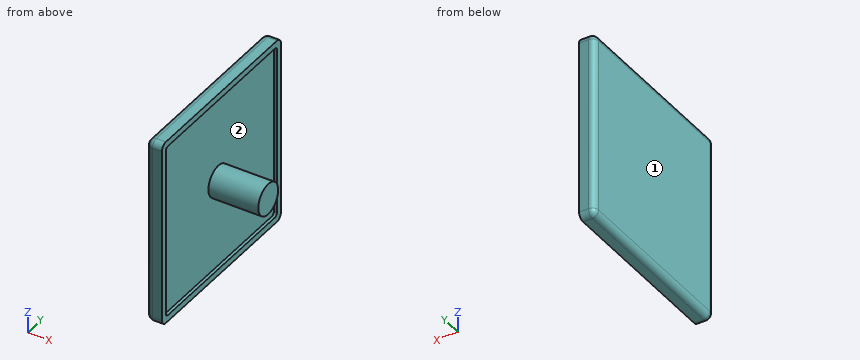
from build123d import *

# Parameters (mm, degrees)
SKETCH2_W           = 30
SKETCH2_H           = 30
BOSS_EXTRUDE1_DEPTH = 2.5
SKETCH3_W           = 28
SKETCH3_H           = 28
CUT_EXTRUDE1_DEPTH  = 0.5
FILLET1_R           = 1
FILLET2_R           = 1
FILLET3_R           = 0.5
SKETCH5_R           = 2.5
BOSS_EXTRUDE2_DEPTH = 8


with BuildPart() as part:
    # Sketch2 → Boss-Extrude1 (new body)
    with BuildSketch(Plane(origin=(0, 0, 0), x_dir=(0, 0, -1), z_dir=(1, 0, 0))):
        with Locations((15, 15)):
            Rectangle(SKETCH2_W, SKETCH2_H)
    extrude(amount=BOSS_EXTRUDE1_DEPTH)

    # Sketch3 → Cut-Extrude1 (cut)
    with BuildSketch(Plane(origin=(2.5, 0, 0), x_dir=(0, 0, -1), z_dir=(1, 0, 0))):
        with Locations((15, 15)):
            Rectangle(SKETCH3_W, SKETCH3_H)
    extrude(amount=-CUT_EXTRUDE1_DEPTH, mode=Mode.SUBTRACT)

    # Fillet1
    fillet1_edges = [part.edges().sort_by_distance(p)[0] for p in [
        (0, 30, -15),
        (0, 15, -30),
        (0, 0, -15),
        (0, 15, 0),
    ]]
    fillet(fillet1_edges, radius=FILLET1_R)

    # Fillet2
    # the kernel refuses this fillet: 1 mm, written as the material it takes off along each edge
    with BuildSketch(Plane(origin=(1, 29, -1), x_dir=(0, 1, 0), z_dir=(0, 0, 1))) as fillet2_piece_1_section:
        Polygon((0, 0), (FILLET2_R, 0), (FILLET2_R, FILLET2_R), (0, FILLET2_R), align=None)
    fillet2_piece_1 = extrude(amount=FILLET2_R, mode=Mode.PRIVATE)
    fillet2_piece_1 = fillet2_piece_1 - Plane(origin=(1, 29, -1), x_dir=(0.7071067811865475, -0.7071067811865475, 0), z_dir=(0, 0, 1)) * Sphere(FILLET2_R, mode=Mode.PRIVATE)
    add(fillet2_piece_1, mode=Mode.SUBTRACT)
    with BuildSketch(Plane(origin=(1, 29, -29), x_dir=(0, 1, 0), z_dir=(0, 0, -1))) as fillet2_piece_2_section:
        Polygon((0, 0), (FILLET2_R, 0), (FILLET2_R, -FILLET2_R), (0, -FILLET2_R), align=None)
    fillet2_piece_2 = extrude(amount=FILLET2_R, mode=Mode.PRIVATE)
    fillet2_piece_2 = fillet2_piece_2 - Plane(origin=(1, 29, -29), x_dir=(0.7071067811865475, -0.7071067811865475, 0), z_dir=(0, 0, -1)) * Sphere(FILLET2_R, mode=Mode.PRIVATE)
    add(fillet2_piece_2, mode=Mode.SUBTRACT)
    with BuildSketch(Plane(origin=(1, 1, -1), x_dir=(0, 0, 1), z_dir=(0, -1, 0))) as fillet2_piece_3_section:
        Polygon((0, 0), (FILLET2_R, 0), (FILLET2_R, FILLET2_R), (0, FILLET2_R), align=None)
    fillet2_piece_3 = extrude(amount=FILLET2_R, mode=Mode.PRIVATE)
    fillet2_piece_3 = fillet2_piece_3 - Plane(origin=(1, 1, -1), x_dir=(0.7071067811865475, 0, -0.7071067811865475), z_dir=(0, -1, 0)) * Sphere(FILLET2_R, mode=Mode.PRIVATE)
    add(fillet2_piece_3, mode=Mode.SUBTRACT)
    with BuildSketch(Plane(origin=(1, 1, -29), x_dir=(0, 0, -1), z_dir=(0, -1, 0))) as fillet2_piece_4_section:
        Polygon((0, 0), (FILLET2_R, 0), (FILLET2_R, -FILLET2_R), (0, -FILLET2_R), align=None)
    fillet2_piece_4 = extrude(amount=FILLET2_R, mode=Mode.PRIVATE)
    fillet2_piece_4 = fillet2_piece_4 - Plane(origin=(1, 1, -29), x_dir=(0.7071067811865475, 0, 0.7071067811865475), z_dir=(0, -1, 0)) * Sphere(FILLET2_R, mode=Mode.PRIVATE)
    add(fillet2_piece_4, mode=Mode.SUBTRACT)
    with BuildSketch(Plane(origin=(1, 30, 0), x_dir=(0, -1, 0), z_dir=(1, 0, 0)), Plane(origin=(1, 0, 0), x_dir=(0, 0, -1), z_dir=(1, 0, 0))) as fillet2_piece_5:
        with BuildLine():
            CenterArc((FILLET2_R, FILLET2_R), FILLET2_R, 180, 90)
            Line((0, FILLET2_R), (0, 0))
            Line((0, 0), (FILLET2_R, 0))
        make_face()
    extrude(amount=4, mode=Mode.SUBTRACT)
    with BuildSketch(Plane(origin=(1, 30, -30), x_dir=(0, -1, 0), z_dir=(1, 0, 0)), Plane(origin=(1, 0, -30), x_dir=(0, 0, 1), z_dir=(1, 0, 0))) as fillet2_piece_6:
        with BuildLine():
            CenterArc((FILLET2_R, -FILLET2_R), FILLET2_R, 90, 90)
            Line((0, -FILLET2_R), (0, 0))
            Line((0, 0), (FILLET2_R, 0))
        make_face()
    extrude(amount=4, mode=Mode.SUBTRACT)

    # Fillet3
    fillet3_edges = [part.edges().sort_by_distance(p)[0] for p in [
        (2.25, 1, -1),
        (2.25, 29, -1),
        (2.25, 29, -29),
        (2.25, 1, -29),
    ]]
    fillet(fillet3_edges, radius=FILLET3_R)

    # Sketch5 → Boss-Extrude2 (add)
    with BuildSketch(Plane(origin=(2, 0, 0), x_dir=(0, 0, -1), z_dir=(1, 0, 0))):
        with Locations((15, 15)):
            Circle(SKETCH5_R)
    extrude(amount=BOSS_EXTRUDE2_DEPTH)


solid = part.part
Geometry check sheet. Reference: the model listing, model coordinates, mm. Face numbers are marked on the shaded views. Coordinates: 2 decimals unless noted, no trailing zeros. Write each loop counter-clockwise with the first axis right and the second up, starting at its lowest first coordinate (ties: lowest second). Pieces come first, ordered by that corner, then holes. Notation, with made-up numbers: (79.5, 62.25) -> (138.5, 62.25) arc R20 cw to (138.5, 84.25) -> close; hole circle Ø1 at (39.25, -39.75). An arc over 180 degrees is marked (long way). One line per question, with ' | ' between items.
1. Cross-section at C-C on x = 7.5. Record the cut outline in (y, z).
Answers:
outline: circle Ø5 at (15, -15)
2. Draft check along Z on the marked faces 1 and 2. Enter one of: +Z half, -Z half, draft (parallel to the pull), parting line (faces both ways), or undercut.
Answers:
face 1: draft | face 2: undercut
3. Cross-section at B-B on z = -7.75. Record the cut outline in (x, y).
Answers:
outline: (0, 1) arc R1 ccw to (1, 0) -> (2.5, 0) -> (2.5, 1) -> (2, 1) -> (2, 29) -> (2.5, 29) -> (2.5, 30) -> (1, 30) arc R1 ccw to (0, 29) -> close
4. Depth check by flat-ended pin: pin 1 Ø6 at (x, y) = (6, 15) entering from -Z. Enter the tip coordinate at first touch or a pass-through.
Answers:
pin 1: stops at z = -17.5
5. Cross-section at A-A on y = 15. Record the cut outline in (x, z), and give its area (3 significant figures).
Answers:
outline: (0, -29) arc R1 ccw to (1, -30) -> (2.5, -30) -> (2.5, -29) -> (2, -29) -> (2, -17.5) -> (10, -17.5) -> (10, -12.5) -> (2, -12.5) -> (2, -1) -> (2.5, -1) -> (2.5, 0) -> (1, 0) arc R1 ccw to (0, -1) -> close | area: 101 mm²
6. Cross-section at D-D on z = -15. Record the cut outline in (x, y), and give its area (3 significant figures).
Answers:
outline: (0, 1) arc R1 ccw to (1, 0) -> (2.5, 0) -> (2.5, 1) -> (2, 1) -> (2, 12.5) -> (10, 12.5) -> (10, 17.5) -> (2, 17.5) -> (2, 29) -> (2.5, 29) -> (2.5, 30) -> (1, 30) arc R1 ccw to (0, 29) -> close | area: 101 mm²
7. Thickness scan on probe 1 along X at (y, z) = (19.5, -12.5); probe 2 along X at (y, z) = (29.5, -25.75); probe 3 along Y at (x, z) = (0.75, -18.25). Record the ranges inside material, lowest first. Write a range as from..to.
Answers:
probe 1: x = 0..2 | probe 2: x = 0.13..2.5 | probe 3: y = 0.03..29.97
